The model under review builds one solid part; all positions refer to its coordinate system, in mm. Face numbers are marked on the shaded views. Give positions to 0.01 mm unless a question says otherwise; leave off trailing zeros. Write each loop counter-clockwise with the first axis right and the second up, starting at its lowest first coordinate (ties: lowest second). Pieces come first, ordered by that corner, then holes.
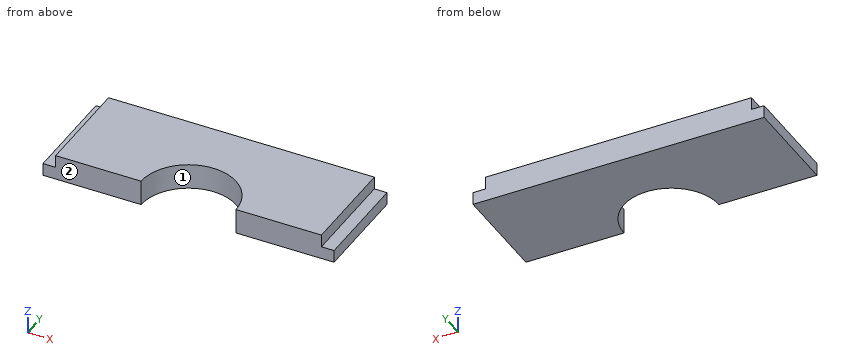
Autodesk Inventor part; units mm, degrees
ref_plane "YZ Plane" through (0, 0, 0) normal (1, 0, 0) x (0, 1, 0)
ref_plane "XZ Plane" through (0, 0, 0) normal (0, 1, 0) x (-1, 0, 0)
ref_plane "XY Plane" through (0, 0, 0) normal (0, 0, 1) x (1, 0, 0)
sketch "Sketch1" plane through (0, 0, 0) normal (0, 1, 0) x (-1, 0, 0)
  line L0 (21, 2) -> (-21, 2)
  line L1 (-21, 2) -> (-21, -2)
  line L2 (-21, -2) -> (21, -2)
  line L3 (21, -2) -> (21, 2)
  line L4 (23, 0) -> (-23, 0)
  line L5 (-23, 0) -> (-23, -2)
  line L6 (-23, -2) -> (23, -2)
  line L7 (23, -2) -> (23, 0)
  point P0 (0, 0)
  dimension "d0" = 42
  dimension "d1" = 4
  dimension "d2" = 21
  dimension "d3" = 2
  dimension "d4" = 2
  dimension "d5" = 46
  dimension "d6" = 2
  dimension "d7" = 2
extrude "Extrusion1" add sketch "Sketch1" along normal blind 16
sketch "Sketch2" plane through (-21, 0, 2) normal (0, 0, 1) x (1, 0, 0)
  circle A0 centre (21, 0) radius 7.5
  dimension "d10" = 15
extrude "Extrusion2" cut sketch "Sketch2" against normal up to next
properties part number "Lid"
1) Consider section D-D, the plane x = 0. Give the boundary of the cut face in (y, z), then the cut area to 3 significant figures.
2) Consider section C-C, the plane y = 11.75. Give the boundary of the cut face in (x, z).
3) Insertion check: pin 1 (2 mm diameter, centred on y = 9, z = 0.5, fed in from +X); pin 2 (1.6 mm diameter, centred on x = 22.5, y = 8.5, fed in from +Z); pin 3 (1 mm diameter, centred on y = 6.5, z = 1.5, fed in from -X). Each pin has a flat end and moves straight along its axis. Give the tip position at first contact, or say it passes through.
4) The part is to be moulded in two halves that separate along X. For the marked faces 1 and 2, say which applies: +X half, -X half, draft (parallel to the pull), parting line (faces both ways), or undercut.
5) To check wall thickness, follow probe 1 along X at (y, z) = (10.25, 0.4); probe 2 along X at (y, z) = (1.25, 1.6); probe 3 along X at (y, z) = (5.25, -1.75). State the ranges of each line that lie inside material, in increasing order.
6) Consider section A-A, the plane y = 4.5. Give the boundary of the cut face in (x, z).
7) Consider section B-B, the plane z = 1.35. Give the boundary of the cut face in (x, y), then the cut area to 3 significant figures.
Answer block:
1. outline: (7.5, -2) - (16, -2) - (16, 2) - (7.5, 2) - close
1. area: 34.0 mm2
2. outline: (-23, -2) - (23, -2) - (23, 0) - (21, 0) - (21, 2) - (-21, 2) - (-21, 0) - (-23, 0) - close
3. pin 1: stops at x = 23
3. pin 2: stops at z = 0
3. pin 3: stops at x = -21
4. face 1: undercut
4. face 2: draft
5. probe 1: x = -21 to 21
5. probe 2: x = -21 to -7.4, 7.4 to 21
5. probe 3: x = -23 to -5.36, 5.36 to 23
6. outline: (-23, -2) - (-6, -2) - (-6, 2) - (-21, 2) - (-21, 0) - (-23, 0) - close; (6, -2) - (23, -2) - (23, 0) - (21, 0) - (21, 2) - (6, 2) - close
7. outline: (-21, 0) - (-7.5, 0) arc R7.5 cw to (7.5, 0) - (21, 0) - (21, 16) - (-21, 16) - close
7. area: 584 mm2
